Autodesk Inventor part; units mm, degrees
ref_plane "YZ Plane" through (0, 0, 0) normal (1, 0, 0) x (0, 1, 0)
ref_plane "XZ Plane" through (0, 0, 0) normal (0, 1, 0) x (-1, 0, 0)
ref_plane "XY Plane" through (0, 0, 0) normal (0, 0, 1) x (1, 0, 0)
sketch "Sketch1" plane through (0, 0, 0) normal (0, 1, 0) x (-1, 0, 0)
  circle A0 centre (0, 0) radius 6.5
  line L0 (0, 0) -> (-32.456, 0) construction
  circle A1 centre (-32.456, 0) radius 4
  arc A2 (-0.9767, -7.9402) -> (-0.9767, 7.9402) centre (0, 0) ccw
  arc A3 (-32.823, 5.9888) -> (-32.823, -5.9888) centre (-32.456, 0) ccw
  line L1 (0, 8) -> (-32.823, 5.9888)
  line L2 (0, -8) -> (-32.823, -5.9888)
  dimension "d0" = 13
  dimension "d1" = 32.456
  dimension "d2" = 8
  dimension "d3" = 16
  dimension "d4" = 12
extrude "Extrusion1" add sketch "Sketch1" along normal blind 3.25 contours L2 A3 L1 A2
properties part number "conex_llantamov"
The model under review builds one solid part; all positions refer to its coordinate system, in mm. Round coordinates to 2 decimals unless told otherwise and drop trailing zeros. Write each loop counter-clockwise with the first axis right and the second up, starting at its lowest first coordinate (ties: lowest second). Pieces come first, ordered by that corner, then holes.
(1) Mouldability with a two-part tool opening along Z and no side actions: class faces 1 (the flat face through (16, 0, 0)), 2 (the cylindrical face through (28.64, 1.6, -1.2)), 3 (the cylindrical face through (38.455, 1.602, -0.127)) as +Z half, -Z half, draft (parallel to the pull), parting line (faces both ways), or undercut.
(2) We need section C-C on z = -4.75. Give the boundary of the cut face in (x, y), and give its area (3 significant figures).
(3) Wall thickness on L1, parallel to Z at x = 0, y = 1.85; L2, parallel to X at y = 2.45, z = -0.75; L3, parallel to X at y = 1, z = 2: over which ranges is each line inside the solid? List them lowest first.
(4) We need section B-B on z = 0. Give the boundary of the cut face in (x, y).
(5) Insertion check: pin 1 (1 mm diameter, centred on x = 3, y = 0.5, fed in from +Z); pin 2 (1.5 mm diameter, centred on x = 12.5, y = 1.5, fed in from +Z); pin 3 (1 mm diameter, centred on y = 1.5, z = 4, fed in from -X); pin 4 (5 mm diameter, centred on x = 32.456, z = 0, fed in from +Y). Each pin has a flat end and moves straight along its axis. Give the tip position at first contact, or say it passes through.
(6) We need section A-A on y = 0.55. Give the boundary of the cut face in (x, z).
(7) We need section D-D on x = 23.5. Give the boundary of the cut face in (y, z).
Findings below:
1. face 1: draft
1. face 2: undercut
1. face 3: parting line
2. outline: (-6.44, 0) - (-4.44, 0) - (-4.44, 3.25) - (-6.44, 3.25) - close; (4.44, 0) - (36.12, 0) - (36.12, 3.25) - (4.44, 3.25) - close
2. area: 109 mm2
3. L1: z = -8 to -6.5, 6.5 to 8
3. L2: x = -7.96 to -6.46, 6.46 to 28.53, 36.39 to 38.41
3. L3: x = -7.75 to -6.18, 6.18 to 28.99, 35.92 to 38.11
4. outline: (-8, 0) - (-6.5, 0) - (-6.5, 3.25) - (-8, 3.25) - close; (6.5, 0) - (28.46, 0) - (28.46, 3.25) - (6.5, 3.25) - close; (36.46, 0) - (38.46, 0) - (38.46, 3.25) - (36.46, 3.25) - close
5. pin 1: stops at z = 7.85
5. pin 2: stops at z = 7.28
5. pin 3: stops at x = -7.19
5. pin 4: passes through
6. outline: (0, -8) - (32.82, -5.99) arc R6 ccw to (32.82, 5.99) - (0, 8) arc R8 ccw to start; hole circle Ø13 at (0, 0); hole circle Ø8 at (32.46, 0)
7. outline: (0, -6.56) - (3.25, -6.56) - (3.25, 6.56) - (0, 6.56) - close
